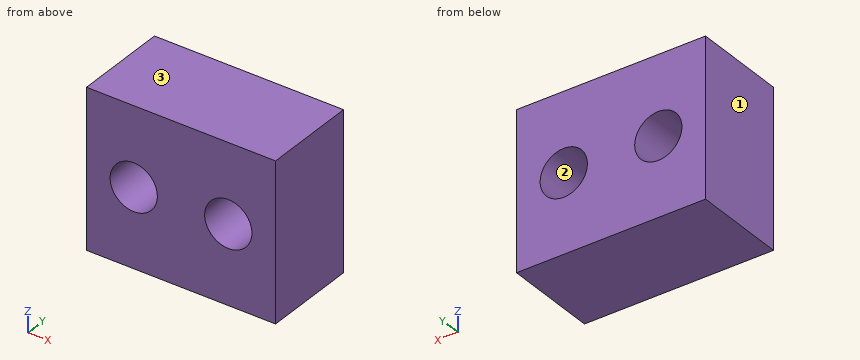
Autodesk Inventor part; units mm, degrees
ref_plane "YZ Plane" through (0, 0, 0) normal (1, 0, 0) x (0, 1, 0)
ref_plane "XZ Plane" through (0, 0, 0) normal (0, 1, 0) x (-1, 0, 0)
ref_plane "XY Plane" through (0, 0, 0) normal (0, 0, 1) x (1, 0, 0)
sketch "Sketch1" plane through (0, 0, 0) normal (0, 1, 0) x (-1, 0, 0)
  line L0 (6, 5) -> (-6, 5)
  line L1 (-6, 5) -> (-6, -5)
  line L2 (-6, -5) -> (6, -5)
  line L3 (6, -5) -> (6, 5)
  line L4 (6, 5) -> (-6, -5) construction
  line L5 (-6, 5) -> (6, -5) construction
  point P0 (0, 0)
  dimension "d0" = 12
  dimension "d1" = 10
extrude "Extrusion1" add sketch "Sketch1" along normal blind 6
sketch "Sketch2" plane through (0, 6, 0) normal (0, 1, 0) x (1, 0, 0)
  line L0 (6, -5) -> (6, 5)
  line L1 (-6, 5) -> (-6, -5)
  line L2 (-6, 0) -> (-3, 0)
  line L3 (6, 0) -> (3, 0)
  circle A0 centre (-3, 0) radius 1.5
  circle A1 centre (3, 0) radius 1.5
  point P0 (0, 0)
  dimension "d4" = 3
  dimension "d5" = 3
  dimension "d6" = 3
  dimension "d7" = 3
extrude "Extrusion2" cut sketch "Sketch2" against normal blind 6
sketch "Sketch3" plane through (0, 0, 0) normal (0, -1, 0) x (1, 0, 0)
  circle A0 centre (-3, 0) radius 1.5
  circle A1 centre (3, 0) radius 1.5
  point P0 (0, 0)
extrude "Extrusion3" add sketch "Sketch3" against normal blind 6
sketch "Sketch4" plane through (0, 0, 0) normal (0, -1, 0) x (1, 0, 0)
  line L0 (-6, -5) -> (-6, 5)
  line L1 (6, 5) -> (6, -5)
  line L2 (-6, 0) -> (-3, 0)
  line L3 (-3, 0) -> (3, 0)
  circle A0 centre (3, 0) radius 1.5
  circle A1 centre (-3, 0) radius 1.5
  point P0 (0, 0)
  dimension "d12" = 3
  dimension "d13" = 6
  dimension "d14" = 3
  dimension "d15" = 3
extrude "Extrusion4" cut sketch "Sketch4" against normal blind 6
properties part number "kolejnicka_ruka_druha_cast"
Geometry check sheet. Reference: the model listing, model coordinates, mm. Face numbers are marked on the shaded views. Round coordinates to 2 decimals unless told otherwise and drop trailing zeros. Loops run counter-clockwise (first coordinate to the right, second up) from the corner with the lowest first, then second, coordinate; pieces in that order, holes last. Notation, with made-up numbers: (-36.5, 88.25) -> (-9.5, 88.25) arc R26 cw to (-9.5, 116.25) -> close; hole circle Ø5 at (-4.5, -25.75). An arc over 180 degrees is marked (long way). Answer as a JSON object with one key per item and string values. Group by question number.
Item 1: Cross-section at C-C, the plane y = 2.6. Record the cut outline in (x, z).
Item 2: Depth check by flat-ended pin: pin 1 Ø5 at (x, z) = (-3, 0) entering from -Y. Enter the tip coordinate at first touch or a pass-through.
Item 3: Release check for a two-part mould opening along X. For the marked faces 1, 2 and 3 record: pulls with the +X half, pulls with the -X half, needs draft (parallel to the pull), parting line crosses it, or undercut.
Item 4: Cross-section at D-D, the plane z = -1.25. Record the cut outline in (x, y).
Item 5: Cross-section at B-B, the plane x = -3. Record the cut outline in (y, z), plus the area to 3 significant figures.
Item 6: Thickness scan on line 1 along X through (y, z) = (3.75, 0); line 2 along Z through (x, y) = (-3, 4); line 3 along X through (y, z) = (3.45, 0.5). Record the ranges inside material, lowest first.
Item 7: Cross-section at A-A, the plane z = 0. Record the cut outline in (x, y), plus the area to 3 significant figures.
Determined:
{
 "1": {"outline": "(-6, -5) -> (6, -5) -> (6, 5) -> (-6, 5) -> close; hole circle Ø3 at (-3, 0); hole circle Ø3 at (3, 0)"},
 "2": {"pin 1": "stops at y = 0"},
 "3": {"face 1": "pulls with the -X half", "face 2": "undercut", "face 3": "needs draft"},
 "4": {"outline": "(-6, 0) -> (-3.83, 0) -> (-3.83, 6) -> (-6, 6) -> close; (-2.17, 0) -> (2.17, 0) -> (2.17, 6) -> (-2.17, 6) -> close; (3.83, 0) -> (6, 0) -> (6, 6) -> (3.83, 6) -> close"},
 "5": {"outline": "(0, -5) -> (6, -5) -> (6, -1.5) -> (0, -1.5) -> close; (0, 1.5) -> (6, 1.5) -> (6, 5) -> (0, 5) -> close", "area": "42.0 mm²"},
 "6": {"line 1": "x = -6 to -4.5, -1.5 to 1.5, 4.5 to 6", "line 2": "z = -5 to -1.5, 1.5 to 5", "line 3": "x = -6 to -4.41, -1.59 to 1.59, 4.41 to 6"},
 "7": {"outline": "(-6, 0) -> (-4.5, 0) -> (-4.5, 6) -> (-6, 6) -> close; (-1.5, 0) -> (1.5, 0) -> (1.5, 6) -> (-1.5, 6) -> close; (4.5, 0) -> (6, 0) -> (6, 6) -> (4.5, 6) -> close", "area": "36.0 mm²"}
}
